Source: CAD feature listing. Evaluate the final solid. Frame: model axes, mm. A direction names the side the tool comes from. Round coordinates to 2 decimals unless told otherwise and drop trailing zeros. Loops run counter-clockwise (first coordinate to the right, second up) from the corner with the lowest first, then second, coordinate; pieces in that order, holes last. Notation, with made-up numbers: (45, 27.25) -> (69, 27.25) arc R14 cw to (69, 44.25) -> close; hole circle Ø2 at (57, 50). An arc over 180 degrees is marked (long way). Write item = value, one per line.
from build123d import *

# Parameters (mm, degrees)
F0_R        = 11.3737467854
F1_DEPTH    = 25.4
F2_R        = 10.5009772193
F3_R        = 10.4902
F4_R        = 10.4902
F5_T1_DEPTH = 25.4
F6_R        = 10.4902
F7_T1_DEPTH = 25.4


# Not quite as in the source:
# - a fillet or chamfer that OpenCascade refuses, or shapes differently, is made with other operations: its cross-section is extruded or revolved along the edge and cut away or added


with BuildPart() as f1:
    # F0 (on Top) → F1 (new body)
    with BuildSketch(Plane.XY):
        with BuildLine():
            ThreePointArc((6.2894283282, 14.6999955177), (13.345564471, 20.5941585441), (15.9889579684, 29.3999910355))
            ThreePointArc((15.9889579684, 29.3999910355), (-8.8058324914, 42.7455555065), (-6.2894283282, 14.6999955177))
            ThreePointArc((-6.2894283282, 14.6999955177), (0, 15.9889579684), (6.2894283282, 14.6999955177))
        make_face()
        with Locations((0, 29.3999910355)):
            Circle(F0_R, mode=Mode.SUBTRACT)
        with BuildLine():
            ThreePointArc((6.2894283282, 14.6999955177), (0, 13.411033067), (-6.2894283282, 14.6999955177))
            ThreePointArc((-6.2894283282, 14.6999955177), (-12.2780666284, 10.2418678368), (-15.5897168926, 3.5507047362))
            ThreePointArc((-15.5897168926, 3.5507047362), (-12.1065325646, -1.6446399909), (-10.8830575897, -7.7787486371))
            ThreePointArc((-10.8830575897, -7.7787486371), (-10.983181349, -9.5652884184), (-11.2822986655, -11.3294533733))
            ThreePointArc((-11.2822986655, -11.3294533733), (0.0583928669, -15.9888513405), (11.3647491723, -11.246744114))
            ThreePointArc((11.3647491723, -11.246744114), (11.6102118149, -3.3482637899), (15.6083251298, 3.467991286))
            ThreePointArc((15.6083251298, 3.467991286), (12.3051770158, 10.209279873), (6.2894283282, 14.6999955177))
        make_face()
        Circle(F0_R, mode=Mode.SUBTRACT)
        with BuildLine():
            ThreePointArc((42.9620322705, -7.778752828), (33.0532173957, 7.0090339191), (15.6083251298, 3.467991286))
            ThreePointArc((15.6083251298, 3.467991286), (15.893514894, 1.7444085615), (15.9889579684, 0))
            ThreePointArc((15.9889579684, 0), (14.7877867471, -6.0801430936), (11.3647491723, -11.246744114))
            ThreePointArc((11.3647491723, -11.246744114), (28.7174828636, -23.6722677221), (42.9620322705, -7.778752828))
        make_face()
        with Locations((26.9730743021, -7.778752828)):
            Circle(F0_R, mode=Mode.SUBTRACT)
        with BuildLine():
            ThreePointArc((-11.2822986655, -11.3294533733), (-15.3584205367, -4.4458627437), (-15.5897168926, 3.5507047362))
            ThreePointArc((-15.5897168926, 3.5507047362), (-42.2304360948, -12.2246113807), (-11.2822986655, -11.3294533733))
        make_face()
        with Locations((-26.8720155582, -7.7787486371)):
            Circle(F0_R, mode=Mode.SUBTRACT)
        with BuildLine():
            ThreePointArc((-10.8830575897, -7.7787486371), (-12.1065325646, -1.6446399909), (-15.5897168926, 3.5507047362))
            ThreePointArc((-15.5897168926, 3.5507047362), (-15.3584205367, -4.4458627437), (-11.2822986655, -11.3294533733))
            ThreePointArc((-11.2822986655, -11.3294533733), (-10.983181349, -9.5652884184), (-10.8830575897, -7.7787486371))
        make_face()
        with BuildLine():
            ThreePointArc((6.2894283282, 14.6999955177), (0, 15.9889579684), (-6.2894283282, 14.6999955177))
            ThreePointArc((-6.2894283282, 14.6999955177), (0, 13.411033067), (6.2894283282, 14.6999955177))
        make_face()
        with BuildLine():
            ThreePointArc((15.9889579684, 0), (15.893514894, 1.7444085615), (15.6083251298, 3.467991286))
            ThreePointArc((15.6083251298, 3.467991286), (11.6102118149, -3.3482637899), (11.3647491723, -11.246744114))
            ThreePointArc((11.3647491723, -11.246744114), (14.7877867471, -6.0801430936), (15.9889579684, 0))
        make_face()
    extrude(amount=F1_DEPTH)

    # F2
    f2_edges = [f1.edges().sort_by_distance(p)[0] for p in [
        (-11.282299, -11.329453, 12.7),
    ]]
    fillet(f2_edges, radius=F2_R)

    # F3
    f3_edges = [f1.edges().sort_by_distance(p)[0] for p in [
        (6.289428, 14.699996, 12.7),
    ]]
    fillet(f3_edges, radius=F3_R)

    # F4
    f4_edges = [f1.edges().sort_by_distance(p)[0] for p in [
        (11.364749, -11.246744, 12.7),
    ]]
    fillet(f4_edges, radius=F4_R)

    # F5: fillet of radius 10.4902 on 1 edges, made by hand

    # F5_s2 → F5_t1 (join)
    with BuildSketch(Plane.XY):
        with BuildLine():
            ThreePointArc((22.2888959377, 7.5086684708), (17.6379410744, 7.1677184148), (13.298783115, 8.8763249477))
            ThreePointArc((13.298783115, 8.8763249477), (14.7043444266, 6.2792540878), (15.6083251298, 3.467991286))
            ThreePointArc((15.6083251298, 3.467991286), (18.6981853725, 5.9023651862), (22.2888959377, 7.5086684708))
        make_face()
    extrude(amount=F5_T1_DEPTH)

    # F6
    f6_edges = [f1.edges().sort_by_distance(p)[0] for p in [
        (-6.289428, 14.699996, 12.7),
    ]]
    fillet(f6_edges, radius=F6_R)

    # F7: fillet of radius 10.4902 on 1 edges, made by hand

    # F7_s2 → F7_t1 (join)
    with BuildSketch(Plane.XY):
        with BuildLine():
            ThreePointArc((-13.298783115, 8.8763249477), (-17.6110780147, 7.1883289802), (-22.2299741232, 7.5215202571))
            ThreePointArc((-22.2299741232, 7.5215202571), (-18.6660423749, 5.9438160297), (-15.5897168926, 3.5507047362))
            ThreePointArc((-15.5897168926, 3.5507047362), (-14.6876450063, 6.3182166063), (-13.298783115, 8.8763249477))
        make_face()
    extrude(amount=F7_T1_DEPTH)


solid = f1.part
1. Section query B-B (y = 0). Return the cut outline in (x, z), then the cut area to 3 significant figures.
Evaluation:
outline = (-40.84, 0) -> (-35.17, 0) -> (-35.17, 25.4) -> (-40.84, 25.4) -> close; (-18.57, 0) -> (-11.37, 0) -> (-11.37, 25.4) -> (-18.57, 25.4) -> close; (11.37, 0) -> (18.68, 0) -> (18.68, 25.4) -> (11.37, 25.4) -> close; (35.27, 0) -> (40.94, 0) -> (40.94, 25.4) -> (35.27, 25.4) -> close
area = 656 mm²
2. Section query A-A (x = 0). Return the cut outline in (y, z), then the cut area to 3 significant figures.
Evaluation:
outline = (-15.99, 0) -> (-11.37, 0) -> (-11.37, 25.4) -> (-15.99, 25.4) -> close; (11.37, 0) -> (18.03, 0) -> (18.03, 25.4) -> (11.37, 25.4) -> close; (40.77, 0) -> (45.39, 0) -> (45.39, 25.4) -> (40.77, 25.4) -> close
area = 403 mm²
3. Section query C-C (y = 22.5). Return the cut outline in (x, z), then the cut area to 3 significant figures.
Evaluation:
outline = (-14.42, 0) -> (-9.04, 0) -> (-9.04, 25.4) -> (-14.42, 25.4) -> close; (9.04, 0) -> (14.42, 0) -> (14.42, 25.4) -> (9.04, 25.4) -> close
area = 273 mm²
4. Line query: probe 1 along Y at (x, z) = (0, 8.5); probe 2 along Y at (x, z) = (-8.5, 8.5); probe 3 along X at (y, z) = (30, 4.5). Output: solid intervals per line, ascending. Write a range as from..to.
Evaluation:
probe_1 = -15.99..-11.37, 11.37..18.03, 40.77..45.39
probe_2 = -15.08..-7.56, 7.56..21.84, 36.96..42.94
probe_3 = -15.98..-11.36, 11.36..15.98
5. Section query D-D (x = 26.5). Return the cut outline in (y, z).
Evaluation:
outline = (-23.76, 0) -> (-19.14, 0) -> (-19.14, 25.4) -> (-23.76, 25.4) -> close; (3.59, 0) -> (8.2, 0) -> (8.2, 25.4) -> (3.59, 25.4) -> close
6. Contact query for flat-ended pins moving along their axis: pin 1 Ø2 at (y, z) = (24, 17.5) entering from -X; pin 2 Ø1 at (y, z) = (-16.5, 14.5) entering from -X; pin 3 Ø6 at (y, z) = (26, 16.5) entering from -X. Output: stop coordinate, or through.
Evaluation:
pin_1 = -15.37
pin_2 = -40.59
pin_3 = -15.98
7. Set-up query: faces 1 (the face through (-7, 11, 25.4)), 2 (the face through (-17.546, 7.198, 12.522)). Return all of +Z, -Z, +X, -X, +Y, -Y with unobstructed straight access to the full face (end or side cutting, diameter ignored); none if empty.
Evaluation:
face_1 = +Z, +X, -X, +Y, -Y
face_2 = +Z, -Z
